```python
from build123d import *

# Parameters (mm, degrees)
SKETCH006_R   = 1
SKETCH006_R_2 = 1.2
SKETCH006_R_3 = 1.491082
PAD002_DEPTH  = 1.6
SKETCH033_W   = 5.831177
SKETCH033_H   = 20.949042
PAD019_DEPTH  = 5.5
PAD021_DEPTH  = 2
SKETCH053_W   = 19.104945
SKETCH053_H   = 22.868039
PAD026_DEPTH  = 2
SKETCH058_W   = 43.228985
SKETCH058_H   = 5.789597
PAD028_DEPTH  = 4.3
SKETCH110_W   = 3.54
SKETCH110_H   = 12.73
PAD057_DEPTH  = 3
FILLET018_R   = 1.7
SKETCH120_W   = 9
SKETCH120_H   = 4.2
PAD060_DEPTH  = 7
SKETCH121_W   = 35
SKETCH121_H   = 18.5
PAD061_DEPTH  = 1.2
SKETCH122_W   = 34.252625
SKETCH122_H   = 5.289647
PAD062_DEPTH  = 2.8


with BuildPart() as part:
    # Sketch006 → Pad002 (new body)
    with BuildSketch(Plane.XY.offset(3)):
        Polygon((30.75, 54.68), (30.75, -28.32), (28.95, -38.82), (26.75, -43.82), (19.75, -43.82), (19.75, -47.52), (-19.75, -47.52), (-19.75, -43.82), (-26.75, -43.82), (-28.95, -38.82), (-30.75, -28.32), (-30.75, 54.68), (-26.5, 54.68), (-26.5, 57.68), (26.5, 57.68), (26.5, 54.68), align=None)
        with Locations((-27.25, -32.12)):
            Circle(SKETCH006_R, mode=Mode.SUBTRACT)
        with Locations((15.75, -32)):
            Circle(SKETCH006_R, mode=Mode.SUBTRACT)
        with Locations((29.1, 50.68)):
            Circle(SKETCH006_R, mode=Mode.SUBTRACT)
        with Locations((-29.1, 50.68)):
            Circle(SKETCH006_R, mode=Mode.SUBTRACT)
        with Locations((-29.1, 5)):
            Circle(SKETCH006_R, mode=Mode.SUBTRACT)
        with Locations((-29.3, 13)):
            Circle(SKETCH006_R_2, mode=Mode.SUBTRACT)
        with Locations((29.3, 13)):
            Circle(SKETCH006_R_2, mode=Mode.SUBTRACT)
        with Locations((29.1, 5)):
            Circle(SKETCH006_R, mode=Mode.SUBTRACT)
        with Locations((-7.25, -45.92)):
            Circle(SKETCH006_R, mode=Mode.SUBTRACT)
        with Locations((-29.1, -25)):
            Circle(SKETCH006_R, mode=Mode.SUBTRACT)
        with Locations((29.1, -25)):
            Circle(SKETCH006_R, mode=Mode.SUBTRACT)
        with Locations((-14.007447, 49.274082)):
            Circle(SKETCH006_R_3, mode=Mode.SUBTRACT)
    extrude(amount=-PAD002_DEPTH)

    # Sketch033 (on Face30 of Pad002) → Pad019 (join)
    with BuildSketch(Plane(origin=(0, 0, 1.4), x_dir=(1, 0, 0), z_dir=(0, 0, -1))):
        with Locations((-22.462421, -27.118268)):
            Rectangle(SKETCH033_W, SKETCH033_H)
    extrude(amount=PAD019_DEPTH)

    # Sketch046 (on Face5 of Pad019) → Pad021 (join)
    with BuildSketch(Plane(origin=(0, 0, 1.4), x_dir=(1, 0, 0), z_dir=(0, 0, -1))):
        Polygon((21.00816, -56.937296), (21.00816, -41.937296), (6.00816, -41.937296), (6.00816, -56.937296), (6.00816, -59.937296), (17.00816, -59.937296), (17.00816, -56.937296), align=None)
    extrude(amount=PAD021_DEPTH)

    # Sketch053 (on Face5 of Pad021) → Pad026 (join)
    with BuildSketch(Plane(origin=(0, 0, 1.4), x_dir=(1, 0, 0), z_dir=(0, 0, -1))):
        with Locations((0.746086, -5.026741)):
            Rectangle(SKETCH053_W, SKETCH053_H)
    extrude(amount=PAD026_DEPTH)

    # Sketch058 (on Face4 of Pad026) → Pad028 (join)
    with BuildSketch(Plane.XY.offset(3)):
        with Locations((-0.757428, -40.205624)):
            Rectangle(SKETCH058_W, SKETCH058_H)
    extrude(amount=PAD028_DEPTH)

    # Sketch110 (on Face5 of Pad028) → Pad057 (join)
    with BuildSketch(Plane(origin=(0, 0, 1.4), x_dir=(1, 0, 0), z_dir=(0, 0, -1))):
        with Locations((20.398529, -31.503779)):
            Rectangle(SKETCH110_W, SKETCH110_H)
    extrude(amount=PAD057_DEPTH)

    # Fillet018
    fillet018_edges = [part.edges().sort_by_distance(p)[0] for p in [
        (18.628529, 25.138779, -0.1),
        (22.168529, 25.138779, -0.1),
        (22.168529, 37.868779, -0.1),
        (18.628529, 37.868779, -0.1),
    ]]
    fillet(fillet018_edges, radius=FILLET018_R)

    # Sketch120 (on Face1 of Fillet018) → Pad060 (join)
    with BuildSketch(Plane(origin=(0, 0, 1.4), x_dir=(1, 0, 0), z_dir=(0, 0, -1))):
        with Locations((-10.558947, 21.91)):
            Rectangle(SKETCH120_W, SKETCH120_H)
    extrude(amount=PAD060_DEPTH)

    # Sketch121 (on Face56 of Pad060) → Pad061 (join)
    with BuildSketch(Plane.XY.offset(3)):
        with Locations((0.75, -5.57)):
            Rectangle(SKETCH121_W, SKETCH121_H)
    extrude(amount=PAD061_DEPTH)

    # Sketch122 (on Face72 of Pad061) → Pad062 (join)
    with BuildSketch(Plane.XY.offset(4.2)):
        with Locations((0.639808, -11.874083)):
            Rectangle(SKETCH122_W, SKETCH122_H)
    extrude(amount=PAD062_DEPTH)


solid = part.part
```
Design review of the part built by this model. Coordinates are the model's own, in mm. A direction names the side the tool comes from. Coordinates: 2 decimals unless noted, no trailing zeros. Order: outer loops, then holes, each group sorted by start corner. A loop starts at its lowest first (then second) coordinate and runs counter-clockwise, first axis right, second up. Notation, with made-up numbers: M -3.5,70 L 51.5,70 A31 ccw 51.5,98 Z; hole C 35.5,-20.5 d7. An arc over 180 degrees is marked long. Answer as a JSON object with one key per item and string values. Group by question number.
1) Wall thickness on L1, parallel to Z at x = -10.5, y = 6; L2, parallel to Z at x = -17.5, y = -42; L3, parallel to Y at x = 1.5, z = -0.5: over which ranges is each line inside the solid? List them lowest first.
2) Mouldability with a two-part tool opening along X and no side actions: class faces 6 (the flat face through (-25.378, 27, -1)), 7 (the cylindrical face through (28.35, 12.27, 2.21)), 8 (the flat face through (11, 59, 1.4)), 9 (the flat face through (17.766, -12, 6)) as pulls with the +X half, pulls with the -X half, needs draft (parallel to the pull), parting line crosses it, or undercut.
3) Add section A-A, the plane y = -45.92. Write out the cut boundary in (x, z).
4) Add section B-B, the plane x = -7.25. Write out the cut boundary in (y, z), then the cut area to 3 significant figures.
5) Tool access review of faces 1 (the flat face through (-11, -24.01, -2)), 2 (the flat face through (14, 41.937, 0)), 3 (the flat face through (18.629, 32, 0)), 4 (the flat face through (20, 31, -1.6)), 5 (the cylindrical face through (28.1, 5, 2.2)): name each direction out of +Z, -Z, +X, -X, +Y, -Y from which nothing blocks a thin tool from reaching the whole face with its end or side.
6) Add section C-C, the plane z = 6. Write out the cut boundary in (x, y), then the cut area to 3 significant figures.
7) Add section D-D, the plane y = 19. Write out the cut boundary in (x, z).
8) For pin 1 (1.3 mm diameter, centred on y = -9, z = 4, fed in from +X); pin 2 (2.5 mm diameter, centred on x = -29.1, y = 50.68, fed in from -Z); pin 3 (3 mm diameter, centred on y = 26, z = -0.5, fed in from -X); pin 4 (1.5 mm diameter, centred on y = -3.5, z = -2.5, fed in from -X), all flat-tipped, find the tip position at first contact; note any pin that passes through.
Computed values:
{
 "1": {"L1": "z = 1.4 to 3", "L2": "z = 1.4 to 7.3", "L3": "y = -6.41 to 16.46"},
 "2": {"face 6": "pulls with the -X half", "face 7": "undercut", "face 8": "needs draft", "face 9": "pulls with the +X half"},
 "3": {"outline": "M -19.75,1.4 L -8.25,1.4 L -8.25,3 L -19.75,3 Z; M -6.25,1.4 L 19.75,1.4 L 19.75,3 L -6.25,3 Z"},
 "4": {"outline": "M -47.52,1.4 L -46.92,1.4 L -46.92,3 L -47.52,3 Z; M -44.92,1.4 L -24.01,1.4 L -24.01,-5.6 L -19.81,-5.6 L -19.81,1.4 L -6.41,1.4 L -6.41,-0.6 L 16.46,-0.6 L 16.46,1.4 L 57.68,1.4 L 57.68,3 L 3.68,3 L 3.68,4.2 L -9.23,4.2 L -9.23,7 L -14.52,7 L -14.52,4.2 L -14.82,4.2 L -14.82,3 L -37.31,3 L -37.31,7.3 L -43.1,7.3 L -43.1,3 L -44.92,3 Z", "area": "302 mm^2"},
 "5": {"face 1": "-Z, +X, -X, -Y", "face 2": "-Z, +X, -X", "face 3": "-Z, -Y", "face 4": "-Z, +X, +Y, -Y", "face 5": "+Z, -Z"},
 "6": {"outline": "M -22.37,-43.1 L 20.86,-43.1 L 20.86,-37.31 L -22.37,-37.31 Z; M -16.49,-14.52 L 17.77,-14.52 L 17.77,-9.23 L -16.49,-9.23 Z", "area": "431 mm^2"},
 "7": {"outline": "M -30.75,1.4 L -25.38,1.4 L -25.38,-4.1 L -19.55,-4.1 L -19.55,1.4 L 30.75,1.4 L 30.75,3 L -30.75,3 Z"},
 "8": {"pin 1": "stops at x = 18.25", "pin 2": "stops at z = 1.4", "pin 3": "stops at x = -25.38", "pin 4": "passes through"}
}
